Can you work these out from the drawing? Everything is in mm from the part's minimum corner. A direction names the side the tool comes from. Give positions to 0.01 mm unless a question says otherwise; leave off trailing zeros. Order: outer loops, then holes, each group sorted by start corner. A loop starts at its lowest first (then second) coordinate and runs counter-clockwise, first axis right, second up. Notation, with made-up numbers: (65, 68) - (78, 68) arc R16 ccw to (78, 83) - close; hole circle Ø6 at (-19.75, 43). An arc over 180 degrees is marked (long way). Write each question's results on one line, items separated by ' | '. Start each with the question number.
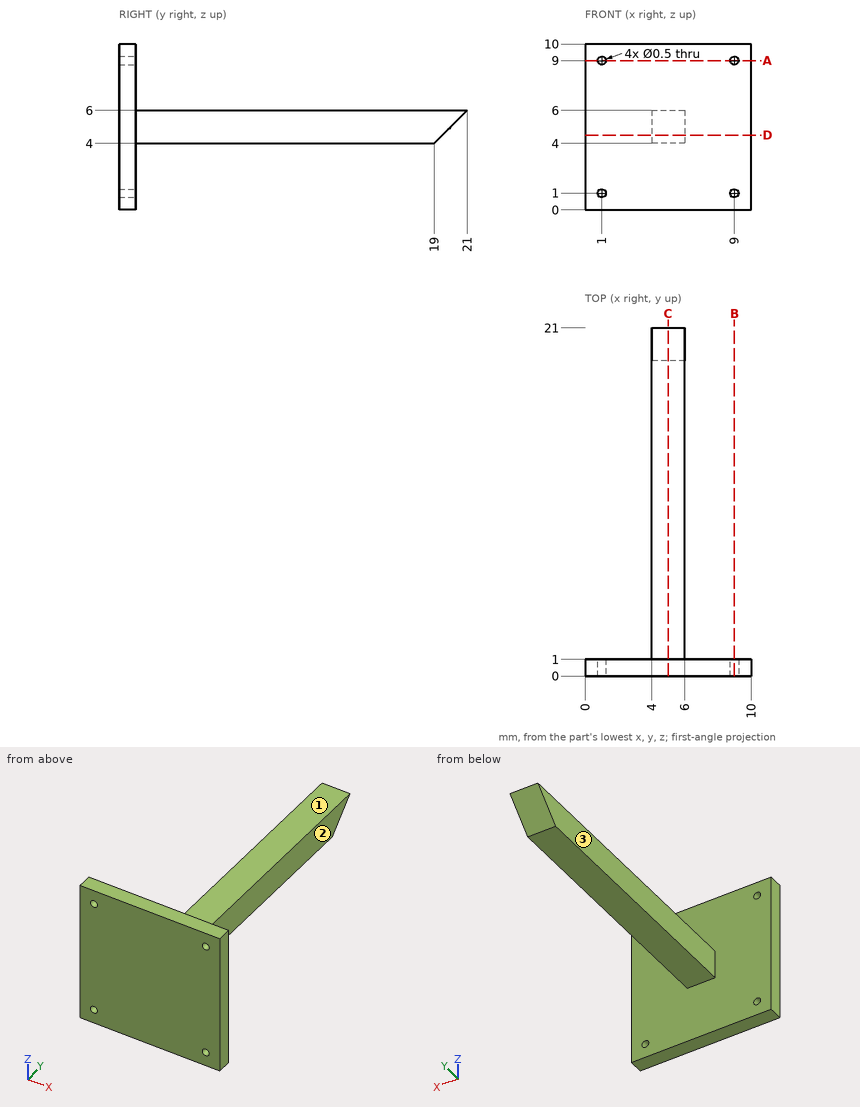
Q1. If we section it at C-C (x = 5): Please give me the cut outline in (y, z), plus the area to 3 significant figures.
Q2. If I drill on probe 1 along Z at (x, y) = (9, 0.35); probe 2 along Y at (x, z) = (6.75, 7.5), over which ranges is the centre line in solid material (lowest first)? Write a range as from..to.
Q3. Which directions (+Z, -Z, +X, -X, +Y, -Y) give clear straight access to the entire face, cutting with the end or side of a thin tool? Please do the marked faces 1, 2 and 3.
Q4. If we section it at D-D (z = 4.5): Please give me the cut outline in (x, y), plus the area to 3 significant figures.
Q5. Will these pins go through, and if not, where does the flat tip stop? P1, Ø0.6, axis at y = 13, z = 5, coming from the +X side; P2, Ø0.6, axis at x = 4.5, y = 8.5, coming from the -Z side; P3, Ø1, axis at y = 16, z = 4.5, coming from the -X side.
Q6. If we section it at A-A (z = 9): Please give me the cut outline in (x, y), plus the area to 3 significant figures.
Q7. If we section it at B-B (x = 9): Please give me the cut outline in (y, z), plus the area to 3 significant figures.
Findings below:
1) outline: (0, 0) - (1, 0) - (1, 4) - (19, 4) - (21, 6) - (1, 6) - (1, 10) - (0, 10) - close | area: 48.0 mm2
2) probe 1: z = 0..0.75, 1.25..8.75, 9.25..10 | probe 2: y = 0..1
3) face 1: +Z, +X, -X, +Y | face 2: +Z, -Z, +X, +Y | face 3: +Z, -Z, -X, +Y
4) outline: (0, 0) - (10, 0) - (10, 1) - (6, 1) - (6, 19.5) - (4, 19.5) - (4, 1) - (0, 1) - close | area: 47.0 mm2
5) P1: stops at x = 6 | P2: stops at z = 4 | P3: stops at x = 4
6) outline: (0, 0) - (0.75, 0) - (0.75, 1) - (0, 1) - close; (1.25, 0) - (8.75, 0) - (8.75, 1) - (1.25, 1) - close; (9.25, 0) - (10, 0) - (10, 1) - (9.25, 1) - close | area: 9.00 mm2
7) outline: (0, 0) - (1, 0) - (1, 0.75) - (0, 0.75) - close; (0, 1.25) - (1, 1.25) - (1, 8.75) - (0, 8.75) - close; (0, 9.25) - (1, 9.25) - (1, 10) - (0, 10) - close | area: 9.00 mm2
